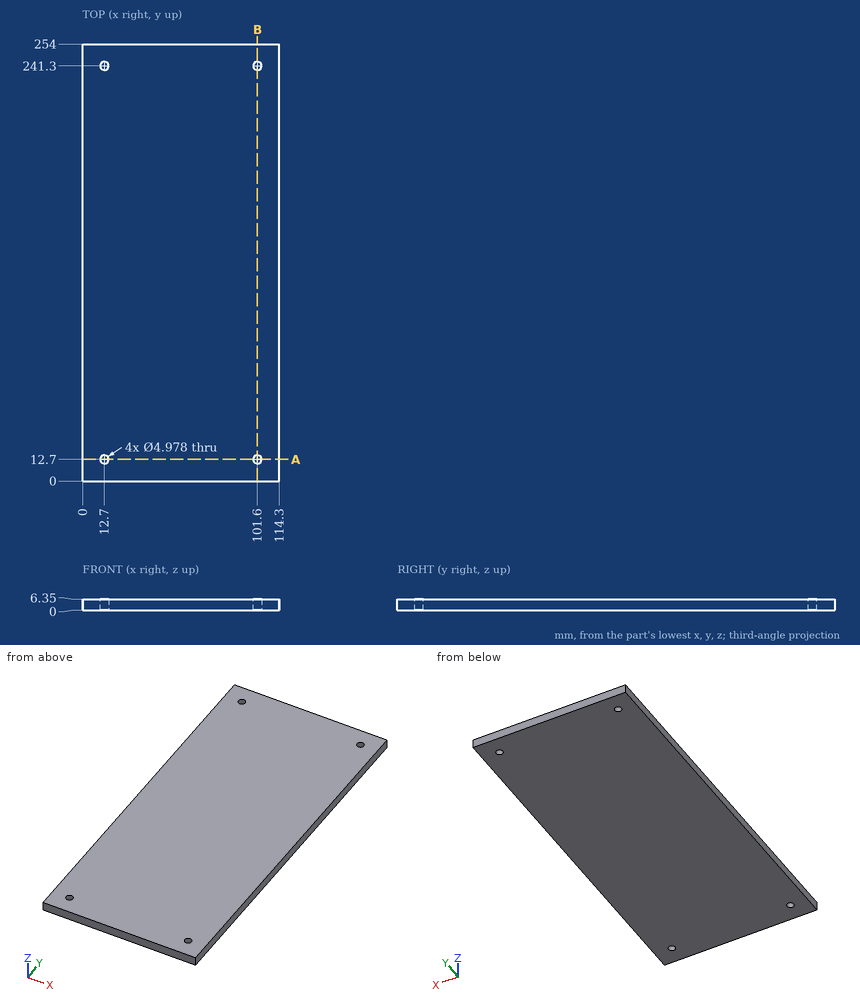
Geometry: see drawing. Coordinates: mm, zero at the bounding-box minimum. Give positions to 0.01 mm unless a question says otherwise; leave off trailing zeros. Order: outer loops, then holes, each group sorted by start corner. A loop starts at its lowest first (then second) coordinate and runs counter-clockwise, first axis right, second up. Notation, with made-up numbers: (9.5, 17) -> (67.5, 17) arc R25 cw to (67.5, 45) -> close; hole circle Ø11 at (-21.75, 13). An arc over 180 degrees is marked (long way). Write item = value, one per line.
Q1. Cut plane B-B, the plane x = 101.6. Output: boundary loops of the cut face in (y, z).
Data:
outline = (0, 0) -> (10.21, 0) -> (10.21, 6.35) -> (0, 6.35) -> close; (15.19, 0) -> (238.81, 0) -> (238.81, 6.35) -> (15.19, 6.35) -> close; (243.79, 0) -> (254, 0) -> (254, 6.35) -> (243.79, 6.35) -> close
Q2. Material intervals for line 1 (X direction, y = 241.3, z = 2); line 2 (Y direction, x = 12.7, z = 3.75); line 3 (X direction, y = 240.5, z = 2.75), sorted ascending. Write a range as from..to.
Data:
line_1 = 0..10.21, 15.19..99.11, 104.09..114.3
line_2 = 0..10.21, 15.19..238.81, 243.79..254
line_3 = 0..10.34, 15.06..99.24, 103.96..114.3
Q3. Cut plane A-A, the plane y = 12.7. Output: boundary loops of the cut face in (x, z).
Data:
outline = (0, 0) -> (10.21, 0) -> (10.21, 6.35) -> (0, 6.35) -> close; (15.19, 0) -> (99.11, 0) -> (99.11, 6.35) -> (15.19, 6.35) -> close; (104.09, 0) -> (114.3, 0) -> (114.3, 6.35) -> (104.09, 6.35) -> close
